from build123d import *

# Parameters (mm, degrees)
SKETCH2_W            = 120
SKETCH2_H            = 43
BOSS_EXTRUDE1_DEPTH  = 38
SKETCH3_W            = 116
SKETCH3_H            = 39
CUT_EXTRUDE1_DEPTH   = 38
BOSS_EXTRUDE2_DEPTH  = 39
SKETCH5_W            = 43
SKETCH5_H            = 38
BOSS_EXTRUDE3_DEPTH  = 2.5
SKETCH6_W            = 2
SKETCH6_H            = 38
BOSS_EXTRUDE4_DEPTH  = 17
SKETCH7_W            = 34
SKETCH7_H            = 38
BOSS_EXTRUDE5_DEPTH  = 18
SKETCH8_W            = 4
SKETCH8_H            = 38
BOSS_EXTRUDE6_DEPTH  = 43
SKETCH9_W            = 18
SKETCH9_H            = 5
CUT_EXTRUDE2_DEPTH   = 41
SKETCH11_W           = 120
SKETCH11_H           = 2
CUT_EXTRUDE3_DEPTH   = 118.5
CUT_EXTRUDE4_DEPTH   = 3
MIRROR4_COPY_1_DEPTH = 3
CUT_EXTRUDE5_START   = -114
SKETCH13_R           = 1
CUT_EXTRUDE5_DEPTH   = 114
SKETCH14_W           = 116
SKETCH14_H           = 2
CUT_EXTRUDE6_DEPTH   = 16.6
SKETCH15_R           = 1.75
CUT_EXTRUDE7_DEPTH   = 1


with BuildPart() as part:
    # Sketch2 → Boss-Extrude1 (new body)
    with BuildSketch(Plane(origin=(0, 0, 0), x_dir=(1, 0, 0), z_dir=(0, 1, 0))):
        Rectangle(SKETCH2_W, SKETCH2_H)
    extrude(amount=BOSS_EXTRUDE1_DEPTH)

    # Sketch3 → Cut-Extrude1 (cut)
    with BuildSketch(Plane(origin=(0, 38, 0), x_dir=(1, 0, 0), z_dir=(0, 1, 0))):
        Rectangle(SKETCH3_W, SKETCH3_H)
    extrude(amount=-CUT_EXTRUDE1_DEPTH, mode=Mode.SUBTRACT)

    # Sketch4 → Boss-Extrude2 (add)
    with BuildSketch(Plane.XY.offset(-19.5)):
        Polygon((-58, 0), (-58, 15), (-38, 0), align=None)
    extrude(amount=BOSS_EXTRUDE2_DEPTH)

    # Sketch5 → Boss-Extrude3 (add)
    with BuildSketch(Plane(origin=(60, 0, 0), x_dir=(0, 0, -1), z_dir=(1, 0, 0))):
        with Locations((0, 19)):
            Rectangle(SKETCH5_W, SKETCH5_H)
    extrude(amount=BOSS_EXTRUDE3_DEPTH)

    # Sketch6 → Boss-Extrude4 (add)
    with BuildSketch(Plane(origin=(0, 0, -21.5), x_dir=(-1, 0, 0), z_dir=(0, 0, -1))):
        with Locations((-61.5, 19)):
            Rectangle(SKETCH6_W, SKETCH6_H)
    extrude(amount=BOSS_EXTRUDE4_DEPTH)

    # Mirror1: part across plane


with BuildPart() as part_1:
    add(part.part)
    add(part.part.mirror(Plane(origin=(0, 0, -38.5), x_dir=(1, 0, 0), z_dir=(0, 0, -1))))

    # Sketch7 → Boss-Extrude5 (add)
    with BuildSketch(Plane(origin=(62.5, 0, 0), x_dir=(0, 0, -1), z_dir=(1, 0, 0))):
        with Locations((38.5, 19)):
            Rectangle(SKETCH7_W, SKETCH7_H)
    extrude(amount=BOSS_EXTRUDE5_DEPTH)

    # Sketch8 → Boss-Extrude6 (add)
    with BuildSketch(Plane.XY.offset(-21.5)):
        with Locations((78.5, 19)):
            Rectangle(SKETCH8_W, SKETCH8_H)
    boss_extrude6 = extrude(amount=BOSS_EXTRUDE6_DEPTH)

    # Sketch9 → Cut-Extrude2 (cut)
    with BuildSketch(Plane.XY.offset(21.5)):
        with Locations((69.5, 27.5)):
            Rectangle(SKETCH9_W, SKETCH9_H)
        with Locations((69.5, 10.5)):
            Rectangle(SKETCH9_W, SKETCH9_H)
    cut_extrude2 = extrude(amount=-CUT_EXTRUDE2_DEPTH, mode=Mode.SUBTRACT)

    # Mirror2: Boss-Extrude6, Cut-Extrude2 across plane
    add(boss_extrude6.mirror(Plane(origin=(0, 0, -38.5), x_dir=(1, 0, 0), z_dir=(0, 0, -1))))
    add(cut_extrude2.mirror(Plane(origin=(0, 0, -38.5), x_dir=(1, 0, 0), z_dir=(0, 0, -1))), mode=Mode.SUBTRACT)

    # Sketch11 → Cut-Extrude3 (cut)
    with BuildSketch(Plane(origin=(80.5, 0, 0), x_dir=(0, 0, -1), z_dir=(1, 0, 0))):
        with Locations((38.5, 1)):
            Rectangle(SKETCH11_W, SKETCH11_H)
    extrude(amount=-CUT_EXTRUDE3_DEPTH, mode=Mode.SUBTRACT)

    # Sketch12 → Cut-Extrude4 (cut)
    with BuildSketch(Plane.XY.offset(21.5)):
        with BuildLine():
            Line((-38, 2), (-49.614835193, 2))
            ThreePointArc((-49.614835193, 2), (-56.018375168, 7.287996976), (-60, 0))
            Line((-60, 0), (-38, 0))
            Line((-38, 0), (-38, 2))
        make_face()
    cut_extrude4 = extrude(amount=-CUT_EXTRUDE4_DEPTH, mode=Mode.SUBTRACT)

    # Mirror3: Cut-Extrude4 across plane
    add(cut_extrude4.mirror(Plane.XY), mode=Mode.SUBTRACT)

    # Mirror4: Cut-Extrude4 across plane
    add(cut_extrude4.mirror(Plane(origin=(0, 0, -38.5), x_dir=(1, 0, 0), z_dir=(0, 0, -1))), mode=Mode.SUBTRACT)

    # Mirror4 copy 1 sketch → Mirror4 copy 1 (cut)
    with BuildSketch(Plane.XY.offset(-55.5)):
        with BuildLine():
            Line((-38, 2), (-49.614835193, 2))
            ThreePointArc((-49.614835193, 2), (-56.018375168, 7.287996976), (-60, 0))
            Line((-60, 0), (-38, 0))
            Line((-38, 0), (-38, 2))
        make_face()
    extrude(amount=-MIRROR4_COPY_1_DEPTH, mode=Mode.SUBTRACT)

    # Sketch13 → Cut-Extrude5 (cut)
    with BuildSketch(Plane.XY.offset(18.5).offset(CUT_EXTRUDE5_START)):
        with Locations((-58, 2)):
            Circle(SKETCH13_R)
    extrude(amount=CUT_EXTRUDE5_DEPTH, mode=Mode.SUBTRACT)

    # Chamfer1
    # the kernel refuses this chamfer: 10 mm, written as the material it takes off along each edge
    with BuildSketch(Plane(origin=(-49.614835193, 2, 38.180669666), x_dir=(-0.41152080336556635, 0.9114003666870882, 0), z_dir=(0, 0, -1))) as chamfer1_piece_1:
        with BuildLine():
            Line((4.024103798, 0), (-2.897424879, 6.010331734))
            Line((-2.897424879, 6.010331734), (-3.079704953, 5.928027573))
            ThreePointArc((-3.079704953, 5.928027573), (-1.554736759, 2.957293148), (-0.182280073, -0.082304161))
            Line((-0.182280073, -0.082304161), (0.082304161, -0.182280073))
            ThreePointArc((0.082304161, -0.182280073), (2.000716354, 0.27264804), (3.968173362, -0.192020276))
            Line((3.968173362, -0.192020276), (4.024103798, 0))
        make_face()
    extrude(amount=19.680669666, mode=Mode.SUBTRACT)

    # Chamfer2
    # the kernel refuses this chamfer: 10 mm, written as the material it takes off along each edge
    with BuildSketch(Plane(origin=(-49.614835193, 2, -38.180669666), x_dir=(0.9996854583228201, -0.0250795617564035, 0), z_dir=(0, 0, 1))) as chamfer2_piece_1:
        with BuildLine():
            Line((6.672267866, 0), (-1.747462586, 3.624884258))
            Line((-1.747462586, 3.624884258), (-1.896145364, 3.491117927))
            ThreePointArc((-1.896145364, 3.491117927), (-0.623209418, 1.920628258), (-0.199937092, -0.005015912))
            Line((-0.199937092, -0.005015912), (0.005015912, -0.199937092))
            ThreePointArc((0.005015912, -0.199937092), (3.339051469, -0.116294632), (6.677283779, -0.199937092))
            Line((6.677283779, -0.199937092), (6.672267866, 0))
        make_face()
    extrude(amount=19.680669666, mode=Mode.SUBTRACT)

    # Chamfer3
    # the kernel refuses this chamfer: 10 mm, written as the material it takes off along each edge
    with BuildSketch(Plane(origin=(-49.614835193, 2, -38.819330334), x_dir=(0.9996854583228201, -0.02507956175640344, 0), z_dir=(0, 0, -1))) as chamfer3_piece_1:
        with BuildLine():
            Line((6.672267866, 0), (-1.747462586, -3.624884258))
            Line((-1.747462586, -3.624884258), (-1.896145364, -3.491117927))
            ThreePointArc((-1.896145364, -3.491117927), (-0.623209418, -1.920628258), (-0.199937092, 0.005015912))
            Line((-0.199937092, 0.005015912), (0.005015912, 0.199937092))
            ThreePointArc((0.005015912, 0.199937092), (3.339051469, 0.116294632), (6.677283779, 0.199937092))
            Line((6.677283779, 0.199937092), (6.672267866, 0))
        make_face()
    extrude(amount=19.680669666, mode=Mode.SUBTRACT)

    # Chamfer4
    # the kernel refuses this chamfer: 10 mm, written as the material it takes off along each edge
    with BuildSketch(Plane(origin=(-49.614835193, 2, -115.180669666), x_dir=(0.9996854583228201, -0.0250795617564035, 0), z_dir=(0, 0, 1))) as chamfer4_piece_1:
        with BuildLine():
            Line((6.672267866, 0), (-1.747462586, 3.624884258))
            Line((-1.747462586, 3.624884258), (-1.896145364, 3.491117927))
            ThreePointArc((-1.896145364, 3.491117927), (-0.623209418, 1.920628258), (-0.199937092, -0.005015912))
            Line((-0.199937092, -0.005015912), (0.005015912, -0.199937092))
            ThreePointArc((0.005015912, -0.199937092), (3.339051469, -0.116294632), (6.677283779, -0.199937092))
            Line((6.677283779, -0.199937092), (6.672267866, 0))
        make_face()
    extrude(amount=19.680669666, mode=Mode.SUBTRACT)

    # Sketch14 → Cut-Extrude6 (cut)
    with BuildSketch(Plane(origin=(0, 38, 0), x_dir=(1, 0, 0), z_dir=(0, 1, 0))):
        with Locations((0, 20.5)):
            Rectangle(SKETCH14_W, SKETCH14_H)
    cut_extrude6 = extrude(amount=-CUT_EXTRUDE6_DEPTH, mode=Mode.SUBTRACT)

    # Mirror5: Cut-Extrude6 across plane
    add(cut_extrude6.mirror(Plane(origin=(0, 0, -38.5), x_dir=(1, 0, 0), z_dir=(0, 0, -1))), mode=Mode.SUBTRACT)

    # Sketch15 → Cut-Extrude7 (cut)
    with BuildSketch(Plane.XY.offset(-21.5)):
        with Locations((70.2, 21.1)):
            Circle(SKETCH15_R)
    cut_extrude7 = extrude(amount=-CUT_EXTRUDE7_DEPTH, mode=Mode.SUBTRACT)

    # Mirror6: Cut-Extrude7 across plane
    add(cut_extrude7.mirror(Plane(origin=(0, 0, -38.5), x_dir=(1, 0, 0), z_dir=(0, 0, -1))), mode=Mode.SUBTRACT)


solid = part_1.part
Read the model definition and answer for the solid it produces. Units are mm, in the model's axes. A direction names the side the tool comes from. Give positions to 0.01 mm unless a question says otherwise; leave off trailing zeros. Write each loop counter-clockwise with the first axis right and the second up, starting at its lowest first coordinate (ties: lowest second). Pieces come first, ordered by that corner, then holes. Notation, with made-up numbers: (-24, -28) - (-11, -28) arc R21 cw to (-11, -8) - close; hole circle Ø2 at (13.5, 68). An arc over 180 degrees is marked (long way). Use CSV: the item, a comma, the result in double quotes. Start each with the question number.
(1) Find section A-A (z = -5.5). Count the separate pieces of the cut face and the enclosed holes in it, plus the area to 3 significant figures.
(2) Find section B-B (x = 40). Give the vertices of the cut face in (y, z).
(3) Given P1, Ø3.5, axis at x = -47, y = 3.5, coming from the +Z side; P2, Ø0.6, axis at x = 77, y = 11.5, coming from the +Z side; P3, Ø4.5, axis at x = 70.2, y = 21.1, coming from the +Z side; P4, Ø1.6, axis at x = 62, z = 0.5, coming from the -Y side, each flat-ended and moving along its own axis, determine where each tip first touches the part or whether it passes through.
(4) For faces 4 (the flat face through (-52, 3, -95.5)), 5 (the flat face through (-52, 3, -58.5)), 6 (the flat face through (78.5, 27, -78)), 7 (the cylindrical face through (68.45, 21.18, -21.99)), determine the directions among +Z, -Z, +X, -X, +Y, -Y from which every point of the face is accessible in a straight line to the end or side of a thin tool.
(5) Consider line 1 along Z through (x, y) = (39, 16.5); line 2 along X through (y, z) = (24.5, -82); line 3 along Z through (x, y) = (-44, 24). Determine where each line is inside the solid, lowest interval first.
(6) Find section D-D (z = -47.5). Give the vertices of the cut face in (x, y), plus the area to 3 significant figures.
(7) Find section C-C (x = 70.2). Give the vertices of the cut face in (y, z).
(8) Determine the mould class of faces 1 (the flat face through (-1, 12, -19.5)), 2 (the flat face through (-47.161, 3.775, 20.021)), 3 (the flat face through (78, 20, 21.5)) for opening direction Z: +Z half, -Z half, draft (parallel to the pull), parting line (faces both ways), or undercut.
Findings below:
1,separate pieces,"3"
1,enclosed holes,"1"
1,area,"489 mm2"
2,outline,"(2, -98.5) - (38, -98.5) - (38, -96.5) - (2, -96.5) - close; (2, -57.5) - (21.4, -57.5) - (21.4, -55.5) - (2, -55.5) - close; (2, -21.5) - (21.4, -21.5) - (21.4, -19.5) - (2, -19.5) - close; (2, 19.5) - (38, 19.5) - (38, 21.5) - (2, 21.5) - close"
3,P1,"z = 21.5"
3,P2,"z = -19.5"
3,P3,"z = -21.5"
3,P4,"y = 2"
4,face 4,"-Z, -Y"
4,face 5,"-Y"
4,face 6,"-Z"
4,face 7,"+Z"
5,line 1,"-98.5 to -96.5, -57.5 to -55.5, -21.5 to -19.5, 19.5 to 21.5"
5,line 2,"-60 to -58, 58 to 62.5, 76.5 to 80.5"
5,line 3,"-98.5 to -96.5, 19.5 to 21.5"
6,outline,"(60.5, 2) - (80.5, 2) - (80.5, 38) - (60.5, 38) - close"
6,area,"720 mm2"
7,outline,"(2, -55.5) - (19.35, -55.5) - (19.35, -54.5) - (22.85, -54.5) - (22.85, -55.5) - (38, -55.5) - (38, -21.5) - (22.85, -21.5) - (22.85, -22.5) - (19.35, -22.5) - (19.35, -21.5) - (2, -21.5) - close"
8,face 1,"undercut"
8,face 2,"draft"
8,face 3,"+Z half"
